The listing builds one solid part. Answer for the finished solid, in the listing's coordinates (mm). Face numbers are marked on the shaded views. Give positions to 0.01 mm unless a question says otherwise; leave off trailing zeros. Order: outer loops, then holes, each group sorted by start corner. A loop starts at its lowest first (then second) coordinate and runs counter-clockwise, first axis right, second up.
```python
from build123d import *

# Parameters (mm, degrees)
SM_START                         = -4
SM_BASE_FLANGE_1_OUTLINE_W       = 400
SM_BASE_FLANGE_1_OUTLINE_H       = 120
SM_BASE_FLANGE_1_DEPTH           = 8
SM_EDGE_FLANGE_1_STRIP_W         = 33.4732
SM_EDGE_FLANGE_1_STRIP_H         = 8
SM_EDGE_FLANGE_1_STRIP_CUT_DEPTH = 400
SM_EDGE_FLANGE_1_DEPTH           = 400
SM_EDGE_FLANGE_2_STRIP_W         = 33.4732
SM_EDGE_FLANGE_2_STRIP_H         = 8
SM_EDGE_FLANGE_2_STRIP_CUT_DEPTH = 400
SM_EDGE_FLANGE_2_DEPTH           = 400


# Read off the part's stored shape, not the designer's step: 基体-法兰1
# Sheet-metal steps are written as plain solids
with BuildPart() as part:
    # 基体-法兰1 outline → 基体-法兰1 (new body)
    with BuildSketch(Plane(origin=(0, 0, 0), x_dir=(1, 0, 0), z_dir=(0, 1, 0)).offset(SM_START)):
        with Locations((0, 60)):
            Rectangle(SM_BASE_FLANGE_1_OUTLINE_W, SM_BASE_FLANGE_1_OUTLINE_H)
    extrude(amount=SM_BASE_FLANGE_1_DEPTH)

    # 边线-法兰1 strip (across the edge) → 边线-法兰1 strip cut (cut)
    with BuildSketch(Plane(origin=(-200, 4, 0), x_dir=(0, 0, -1), z_dir=(1, 0, 0))):
        with Locations((-8, -4)):
            Rectangle(SM_EDGE_FLANGE_1_STRIP_W, SM_EDGE_FLANGE_1_STRIP_H)
    extrude(amount=SM_EDGE_FLANGE_1_STRIP_CUT_DEPTH, mode=Mode.SUBTRACT)

    # 边线-法兰1 section (across the edge) → 边线-法兰1 (add)
    with BuildSketch(Plane(origin=(-200, 4, 0), x_dir=(0, 0, -1), z_dir=(1, 0, 0))):
        with BuildLine():
            Line((0, 0.7366), (0, 12))
            Line((0, 12), (8, 12))
            Line((8, 12), (8, 0.7366))
            ThreePointArc((8, 0.7366), (8.215745145, 0.215745145), (8.7366, 0))
            Line((8.7366, 0), (8.7366, -8))
            ThreePointArc((8.7366, -8), (2.558890895, -5.441109105), (0, 0.7366))
        make_face()
    extrude(amount=SM_EDGE_FLANGE_1_DEPTH)

    # 边线-法兰2 strip (across the edge) → 边线-法兰2 strip cut (cut)
    with BuildSketch(Plane(origin=(200, 4, -120), x_dir=(0, 0, 1), z_dir=(-1, 0, 0))):
        with Locations((-8, -4)):
            Rectangle(SM_EDGE_FLANGE_2_STRIP_W, SM_EDGE_FLANGE_2_STRIP_H)
    extrude(amount=SM_EDGE_FLANGE_2_STRIP_CUT_DEPTH, mode=Mode.SUBTRACT)

    # 边线-法兰2 section (across the edge) → 边线-法兰2 (add)
    with BuildSketch(Plane(origin=(200, 4, -120), x_dir=(0, 0, 1), z_dir=(-1, 0, 0))):
        with BuildLine():
            Line((0, 0.7366), (0, 12))
            Line((0, 12), (8, 12))
            Line((8, 12), (8, 0.7366))
            ThreePointArc((8, 0.7366), (8.215745145, 0.215745145), (8.7366, 0))
            Line((8.7366, 0), (8.7366, -8))
            ThreePointArc((8.7366, -8), (2.558890895, -5.441109105), (0, 0.7366))
        make_face()
    extrude(amount=SM_EDGE_FLANGE_2_DEPTH)


solid = part.part
```
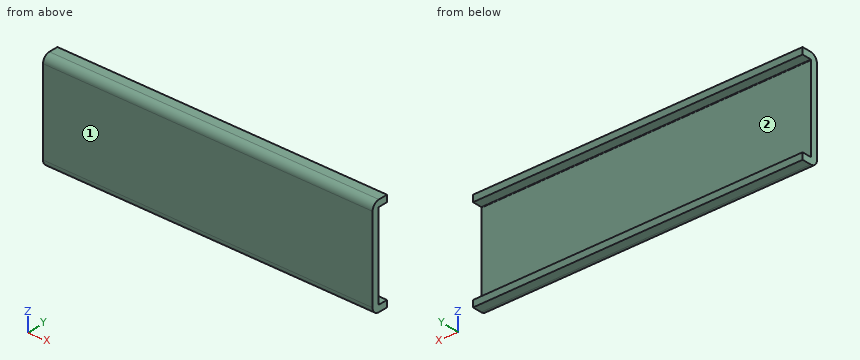
1) Find section C-C (z = -26.5). Write down the section's boundary in (x, y).
Geometry says:
outline: (-200, -4) - (200, -4) - (200, 4) - (-200, 4) - close
2) Find section B-B (x = 112.5). Write down the section's boundary in (y, z).
Geometry says:
outline: (-4, -111.26) arc R8.74 ccw to (4.74, -120) - (16, -120) - (16, -112) - (4.74, -112) arc R0.74 cw to (4, -111.26) - (4, -8.74) arc R0.74 cw to (4.74, -8) - (16, -8) - (16, 0) - (4.74, 0) arc R8.74 ccw to (-4, -8.74) - close
3) For a pull along Z with two mould halves and no side action, classify the marked faces 1 and 2 as +Z half, -Z half, draft (parallel to the pull), parting line (faces both ways), or undercut.
Geometry says:
face 1: draft
face 2: undercut
4) Find section A-A (y = 9). Write down the section's boundary in (x, z), then the cut area to 3 significant figures.
Geometry says:
outline: (-200, -120) - (200, -120) - (200, -112) - (-200, -112) - close; (-200, -8) - (200, -8) - (200, 0) - (-200, 0) - close
area: 6,400 mm2
5) Given P1, Ø8, axis at x = 122.5, z = -92.5, coming from the +Y side, flat-ended and moving along its own axis, determine where the tip first touches the part or whether it passes through.
Geometry says:
P1: stops at y = 4
6) Straight lines are drawn through the part: probe 1 along Z at (x, y) = (-55, 9.5); probe 2 along Y at (x, z) = (93, -54); probe 3 along Z at (x, y) = (19.5, 3.75). For each, find the intervals that lie inside material, in ascending order.
Geometry says:
probe 1: z = -120 to -112, -8 to 0
probe 2: y = -4 to 4
probe 3: z = -119.94 to -0.06
